Build history of the part. All positions in model axes, mm. A direction names the side the tool comes from. Coordinates: 2 decimals unless noted, no trailing zeros. Order: outer loops, then holes, each group sorted by start corner. A loop starts at its lowest first (then second) coordinate and runs counter-clockwise, first axis right, second up. Notation, with made-up numbers: (17, 12.5) - (58, 12.5) arc R23 cw to (58, 21.5) - close; hole circle Ø10 at (41.25, 66). An arc over 180 degrees is marked (long way). One line per item, written item: value.
from build123d import *

# Parameters (mm, degrees)
BASE_W                 = 120
BASE_H                 = 25
BASE_EXT_DEPTH         = 10
SKETCH3_R              = 5.5
LED_BOTTOM_CUT_DEPTH   = 65.13752525
LED_FOR_TOP_ROW_R      = 5.5
LED_TOP_CUT_DEPTH      = 66.86811155
SKETCH5_W              = 120
SKETCH5_H              = 25
SKETCH5_W_2            = 116
SKETCH5_H_2            = 21
WIRE_BOX_RIM_DEPTH     = 5
SKETCH6_W              = 6
SKETCH6_H              = 10
SUPPORT_SPACERS_DEPTH  = 5
SKETCH8_R              = 1.75
M3_SCREW_CUT_DEPTH     = 64.097147321
WIRE_CUT_OUT_RX        = 2.5
WIRE_CUT_OUT_RY        = 2
WIRE_CUT_OUT_CUT_DEPTH = 2
FILLET1_R              = 1
FILLET2_R              = 1
FILLET3_R              = 2
FILLET4_R              = 2
FILLET5_R              = 2
FILLET6_R              = 2
CUT_EXTRUDE5_DEPTH     = 3.5


with BuildPart() as part:
    # Base → Base EXT (new body)
    with BuildSketch(Plane(origin=(0, 0, 0), x_dir=(1, 0, 0), z_dir=(0, 1, 0))):
        Rectangle(BASE_W, BASE_H)
    extrude(amount=BASE_EXT_DEPTH)

    # Sketch3 → LED bottom CUT (cut, through all)
    with BuildSketch(Plane(origin=(0, 13.001715818, 6.062799655), x_dir=(1, 0, 0), z_dir=(0, 0.9063077870366496, 0.4226182617407003))):
        with Locations(Location((-45, 1.897335279, 0), (0, 0, 270))):
            Circle(SKETCH3_R)
        with Locations(Location((0, 1.897335279, 0), (0, 0, 270))):
            Circle(SKETCH3_R)
        with Locations(Location((45, 1.897335279, 0), (0, 0, 270))):
            Circle(SKETCH3_R)
    extrude(amount=-LED_BOTTOM_CUT_DEPTH, mode=Mode.SUBTRACT)

    # LED for Top Row → LED top CUT (cut, through all)
    with BuildSketch(Plane(origin=(0, 9.162978163, 13.086089), x_dir=(1, 0, 0), z_dir=(0, 0.5735764363510444, 0.819152044288993))):
        with Locations(Location((-23.903258736, 8.521814989, 0), (0, 0, 270))):
            Circle(LED_FOR_TOP_ROW_R)
        with Locations(Location((23.903258736, 8.521814989, 0), (0, 0, 270))):
            Circle(LED_FOR_TOP_ROW_R)
    extrude(amount=-LED_TOP_CUT_DEPTH, mode=Mode.SUBTRACT)

    # Sketch5 → Wire Box Rim (add)
    with BuildSketch(Plane(origin=(0, 10, 0), x_dir=(1, 0, 0), z_dir=(0, 1, 0))):
        Rectangle(SKETCH5_W, SKETCH5_H)
        Rectangle(SKETCH5_W_2, SKETCH5_H_2, mode=Mode.SUBTRACT)
    extrude(amount=WIRE_BOX_RIM_DEPTH)

    # Sketch6 → Support Spacers (add)
    with BuildSketch(Plane(origin=(0, 10, 0), x_dir=(1, 0, 0), z_dir=(0, 1, 0))):
        with Locations((-12, 0)):
            Rectangle(SKETCH6_W, SKETCH6_H)
        with Locations((12, 0)):
            Rectangle(SKETCH6_W, SKETCH6_H)
    extrude(amount=SUPPORT_SPACERS_DEPTH)

    # Sketch8 → M3 Screw CUT (cut, through all)
    with BuildSketch(Plane(origin=(0, 15, 0), x_dir=(1, 0, 0), z_dir=(0, 1, 0))):
        with Locations(Location((12, 0, 0), (0, 0, 270))):
            Circle(SKETCH8_R)
        with Locations(Location((-12, 0, 0), (0, 0, 270))):
            Circle(SKETCH8_R)
    extrude(amount=-M3_SCREW_CUT_DEPTH, mode=Mode.SUBTRACT)

    # Wire cut out → Wire cut out CUT (cut)
    with BuildSketch(Plane(origin=(0, 0, -12.5), x_dir=(-1, 0, 0), z_dir=(0, 0, -1))):
        with Locations(Location((0, 15), (0, 0, 180))):
            Ellipse(WIRE_CUT_OUT_RX, WIRE_CUT_OUT_RY)
    extrude(amount=-WIRE_CUT_OUT_CUT_DEPTH, mode=Mode.SUBTRACT)

    # Fillet1
    fillet1_edges = [part.edges().sort_by_distance(p)[0] for p in [
        (2.5, 15, -11.5),
    ]]
    fillet(fillet1_edges, radius=FILLET1_R)

    # Fillet2
    fillet2_edges = [part.edges().sort_by_distance(p)[0] for p in [
        (-2.5, 15, -11.5),
    ]]
    fillet(fillet2_edges, radius=FILLET2_R)

    # Fillet3
    fillet3_edges = [part.edges().sort_by_distance(p)[0] for p in [
        (-60, 7.5, -12.5),
    ]]
    fillet(fillet3_edges, radius=FILLET3_R)

    # Fillet4
    fillet4_edges = [part.edges().sort_by_distance(p)[0] for p in [
        (60, 7.5, -12.5),
    ]]
    fillet(fillet4_edges, radius=FILLET4_R)

    # Fillet5
    fillet5_edges = [part.edges().sort_by_distance(p)[0] for p in [
        (60, 7.5, 12.5),
    ]]
    fillet(fillet5_edges, radius=FILLET5_R)

    # Fillet6
    fillet6_edges = [part.edges().sort_by_distance(p)[0] for p in [
        (-60, 7.5, 12.5),
    ]]
    fillet(fillet6_edges, radius=FILLET6_R)

    # M3 Nut → Cut-Extrude5 (cut)
    with BuildSketch(Plane.XZ):
        Polygon((-12, 3.175426481), (-14.75, 1.58771324), (-14.75, -1.58771324), (-12, -3.175426481), (-9.25, -1.58771324), (-9.25, 1.58771324), align=None)
        Polygon((9.25, 1.58771324), (12, 3.175426481), (14.75, 1.58771324), (14.75, -1.58771324), (12, -3.175426481), (9.25, -1.58771324), align=None)
    extrude(amount=-CUT_EXTRUDE5_DEPTH, mode=Mode.SUBTRACT)


solid = part.part
1. 3-axis set-ups, long thin cutter, end or side, ignore diameter. For faces 1 (the face through (-39.547, 5.358, -0.385)), 2 (the face through (13.394, 1.726, -2.37)), 3 (the face through (-12, 12, 5)): which of +Z, -Z, +X, -X, +Y, -Y reach the whole face in a straight line?
Values found:
face 1: none
face 2: -Y
face 3: +Y
2. Flat gauge pins, fed straight in: P1, Ø10.5, axis at x = 1.5, z = 1, coming from the +Y side; P2, Ø6, axis at x = -12, z = -1.5, coming from the -Y side; P3, Ø1.6, axis at x = 12.5, z = 1, coming from the -Y side. Where does each tip first touch, or does it go through?
Values found:
P1: stops at y = 10
P2: stops at y = 0
P3: stops at y = 3.5
3. Band-saw the part on C-C, the plane y = 7. Count the separate pieces of the cut face and the enclosed holes in it, and give its area (3 significant figures).
Values found:
separate pieces: 1
enclosed holes: 5
area: 2,350 mm2
4. Two-plate mould, pull along Z, no slides. Class faces 4 (the face through (-58, 12, 0)), 5 (the face through (-1, 7, 12.5)), 6 (the face through (60, 7, 0)): pulls with the +Z half, pulls with the -Z half, needs draft (parallel to the pull), parting line crosses it, or undercut.
Values found:
face 4: undercut
face 5: pulls with the +Z half
face 6: needs draft
5. Band-saw the part on B-B, the plane x = -33.5. Give the cut face in (y, z), and give its area (3 significant figures).
Values found:
outline: (0, -12.5) - (15, -12.5) - (15, -10.5) - (10, -10.5) - (10, 10.5) - (15, 10.5) - (15, 12.5) - (0, 12.5) - close
area: 270 mm2
6. Probe line 1 along X through (y, z) = (10.75, 0); line 2 along X through (y, z) = (11.75, 2.25); line 3 along Z through (x, y) = (19, 12.5). List the from-to ranges inside material, lowest first.
Values found:
line 1: x = -60 to -58, -15 to -13.75, -10.25 to -9, 9 to 10.25, 13.75 to 15, 58 to 60
line 2: x = -60 to -58, -15 to -9, 9 to 15, 58 to 60
line 3: z = -12.5 to -10.5, 10.5 to 12.5
7. Band-saw the part on A-A, the plane x = 43. Give the cut face in (y, z), and give its area (3 significant figures).
Values found:
outline: (0, -12.5) - (15, -12.5) - (15, -10.5) - (10, -10.5) - (10, -3.08) - (0, -7.75) - close; (0, 3.56) - (10, 8.22) - (10, 10.5) - (15, 10.5) - (15, 12.5) - (0, 12.5) - close
area: 157 mm2
